Verification items for this drawing (mm, ordinates from the low corner). A direction names the side the tool comes from. Coordinates: 2 decimals unless noted, no trailing zeros. Order: outer loops, then holes, each group sorted by start corner. A loop starts at its lowest first (then second) coordinate and runs counter-clockwise, first axis right, second up. Notation, with made-up numbers: M 85,54.5 L 144,54.5 A18 cw 144,86.5 Z; hole C 43.5,4 d2. An arc over 180 degrees is marked long. Answer as a JSON object with one key per item and string values. Group by question number.
(1) Access from +Z, -Z, +X, -X, +Y, -Y to the whole of each face (thin tool, end or side, straight path). Record for the marked faces 1, 2 and 3.
(2) Cross-section at D-D (y = 32). Enter the section's corners in (x, z) (3 decimals).
(3) Mould release check, pull along X, two halves, no side actions. Record for the marked faces 4, 5, 6 and 7: released by +X, released by -X, zero draft, split by the parting line, or undercut.
(4) Material ranges on line 1 (Z direction, x = 6.75, y = 23); line 2 (Z direction, x = 10.5, y = 29); line 3 (X direction, y = 13, z = 22.5), recorded low to high.
(5) Cross-section at B-B (y = 24). Enter the section's corners in (x, z), plus the area to 3 significant figures.
(6) Cross-section at C-C (z = 27). Enter the section's corners in (x, y) (3 decimals).
(7) Cross-section at A-A (y = 12.7). Enter the section's corners in (x, z).
(8) Gauge pin test, flat ends, axial feed: pin 1 Ø5.5 at (x, y) = (9, 15.5) entering from +Z; pin 2 Ø2 at (x, y) = (13, 27.5) entering from -Z; pin 3 Ø5.5 at (x, y) = (12.5, 14) entering from -Z; pin 4 Ø3 at (x, z) = (15.5, 16.5) entering from -Y. Record the tip position at first contact, or that the pin passes through.
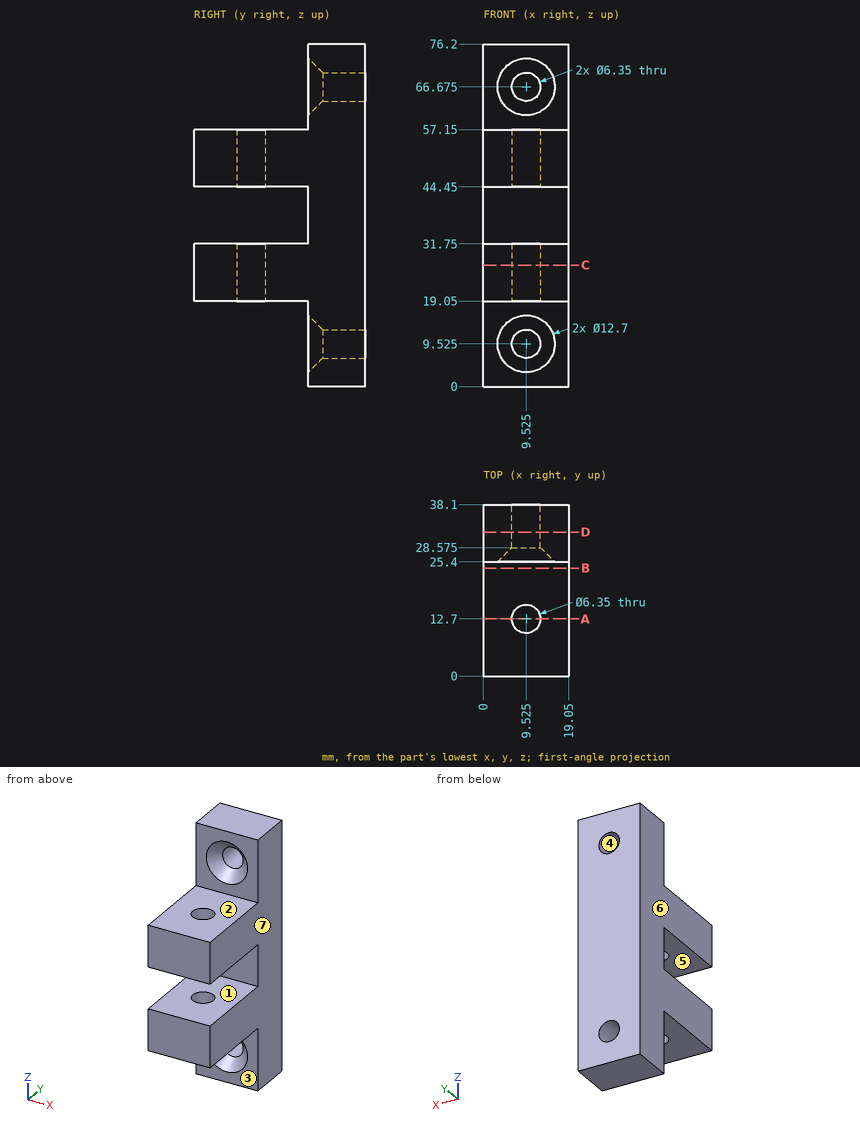
Taken from the geometry:
{
 "1": {"face 1": "+X, -X, -Y", "face 2": "+Z, +X, -X, -Y", "face 3": "-Z, +X, -X, -Y"},
 "2": {"outline": "M 0,0 L 19.05,0 L 19.05,76.2 L 0,76.2 Z; hole C 9.525,9.525 d6.35; hole C 9.525,66.675 d6.35"},
 "3": {"face 4": "undercut", "face 5": "zero draft", "face 6": "released by -X", "face 7": "released by +X"},
 "4": {"line 1": "z = 19.05 to 31.75, 44.45 to 57.15", "line 2": "z = 0 to 6.5, 12.55 to 63.65, 69.7 to 76.2", "line 3": "x = 0 to 6.36, 12.69 to 19.05"},
 "5": {"outline": "M 0,19.05 L 19.05,19.05 L 19.05,31.75 L 0,31.75 Z; M 0,44.45 L 19.05,44.45 L 19.05,57.15 L 0,57.15 Z", "area": "484 mm²"},
 "6": {"outline": "M 0,0 L 19.05,0 L 19.05,38.1 L 0,38.1 Z; hole C 9.525,12.7 d6.35"},
 "7": {"outline": "M 0,19.05 L 6.35,19.05 L 6.35,31.75 L 0,31.75 Z; M 0,44.45 L 6.35,44.45 L 6.35,57.15 L 0,57.15 Z; M 12.7,19.05 L 19.05,19.05 L 19.05,31.75 L 12.7,31.75 Z; M 12.7,44.45 L 19.05,44.45 L 19.05,57.15 L 12.7,57.15 Z"},
 "8": {"pin 1": "stops at z = 57.15", "pin 2": "stops at z = 0", "pin 3": "stops at z = 19.05", "pin 4": "stops at y = 25.4"}
}
